Input: part model. Units: mm. Frame: model coordinates. Face numbers are marked on the shaded views. Coordinates: 2 decimals unless noted, no trailing zeros. Write each loop counter-clockwise with the first axis right and the second up, starting at its lowest first coordinate (ties: lowest second). Pieces come first, ordered by that corner, then holes.
1) Section query B-B (z = 0.4). Output: boundary loops of the cut face in (x, y), then the cut area to 3 significant figures.
2) Draft query along X for the marked faces 1 and 2. Return one class per face: pulls with the +X half, pulls with the -X half, needs draft (parallel to the pull), parting line crosses it, or undercut.
3) Section query C-C (x = 15). Output: boundary loops of the cut face in (y, z).
4) Section query A-A (y = 8.5). Output: boundary loops of the cut face in (x, z).
5) Line query: L1, parallel to X at y = 5, z = 1.55; L2, parallel to Y at x = 14, z = 0.25. Output: solid intervals per line, ascending.
6) Section query D-D (x = 19.25). Output: boundary loops of the cut face in (y, z).
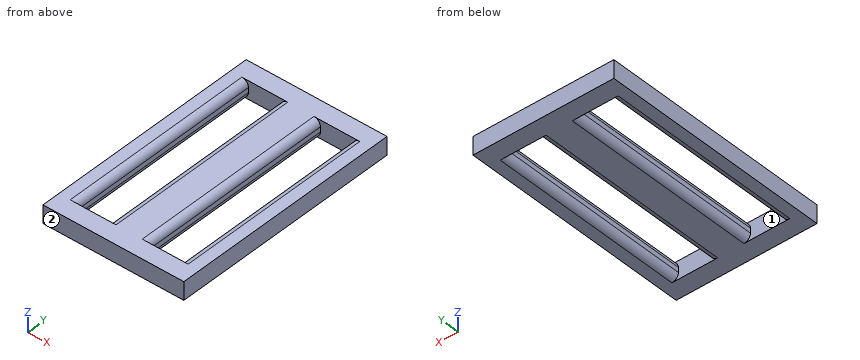
from build123d import *

# Parameters (mm, degrees)
SKETCH1_W           = 5
SKETCH1_H           = 30
BOSS_EXTRUDE1_DEPTH = 2.75
FILLET1_R           = 1


with BuildPart() as part:
    # Sketch1 → Boss-Extrude1 (new body)
    with BuildSketch(Plane.XY):
        Polygon((0, 30), (0, 32.75), (21.5, 32.75), (21.5, 30), (21.5, 0), (21.5, -2.75), (0, -2.75), (0, 0), align=None)
        with Locations((5.25, 15)):
            Rectangle(SKETCH1_W, SKETCH1_H, mode=Mode.SUBTRACT)
        with Locations((16.25, 15)):
            Rectangle(SKETCH1_W, SKETCH1_H, mode=Mode.SUBTRACT)
    extrude(amount=BOSS_EXTRUDE1_DEPTH)

    # Fillet1
    fillet1_edges = [part.edges().sort_by_distance(p)[0] for p in [
        (2.75, 15, 0),
        (7.75, 15, 0),
        (2.75, 15, 2.75),
        (7.75, 15, 2.75),
        (13.75, 15, 0),
        (18.75, 15, 0),
        (13.75, 15, 2.75),
        (18.75, 15, 2.75),
    ]]
    fillet(fillet1_edges, radius=FILLET1_R)


solid = part.part
Answer:
1. outline: (0, -2.75) - (21.5, -2.75) - (21.5, 32.75) - (0, 32.75) - close; hole (2.55, 0) - (7.95, 0) - (7.95, 30) - (2.55, 30) - close; hole (13.55, 0) - (18.95, 0) - (18.95, 30) - (13.55, 30) - close
1. area: 439 mm2
2. face 1: undercut
2. face 2: needs draft
3. outline: (-2.75, 0) - (0, 0) - (0, 2.75) - (-2.75, 2.75) - close; (30, 0) - (32.75, 0) - (32.75, 2.75) - (30, 2.75) - close
4. outline: (0, 0) - (1.75, 0) arc R1 ccw to (2.75, 1) - (2.75, 1.75) arc R1 ccw to (1.75, 2.75) - (0, 2.75) - close; (7.75, 1) arc R1 ccw to (8.75, 0) - (12.75, 0) arc R1 ccw to (13.75, 1) - (13.75, 1.75) arc R1 ccw to (12.75, 2.75) - (8.75, 2.75) arc R1 ccw to (7.75, 1.75) - close; (18.75, 1) arc R1 ccw to (19.75, 0) - (21.5, 0) - (21.5, 2.75) - (19.75, 2.75) arc R1 ccw to (18.75, 1.75) - close
5. L1: x = 0 to 2.75, 7.75 to 13.75, 18.75 to 21.5
5. L2: y = -2.75 to 0, 30 to 32.75
6. outline: (-2.75, 0) - (0, 0) - (0, 0.13) - (30, 0.13) - (30, 0) - (32.75, 0) - (32.75, 2.75) - (30, 2.75) - (30, 2.62) - (0, 2.62) - (0, 2.75) - (-2.75, 2.75) - close
